```python
from build123d import *

# Parameters (mm, degrees)
F0_R     = 70
F1_DEPTH = 16
F2_R     = 31.12
F3_DEPTH = 16.001
F4_R     = 3.15
F4_R_2   = 8
F4_R_3   = 4
F5_DEPTH = 16.001
F6_R     = 45
F7_DEPTH = 2
F8_R     = 60
F8_R_2   = 58
F9_DEPTH = 2


with BuildPart() as f1:
    # F0 (on Top) → F1 (new body)
    with BuildSketch(Plane.XY):
        Circle(F0_R)
    extrude(amount=F1_DEPTH)

    # F2 (on face) → F3 (cut, through all)
    with BuildSketch(Plane.XY.offset(16)):
        Circle(F2_R)
    extrude(amount=-F3_DEPTH, mode=Mode.SUBTRACT)

    # F4 (on face) → F5 (cut, through all)
    with BuildSketch(Plane(origin=(0, 0, 0), x_dir=(1, 0, 0), z_dir=(0, 0, -1))):
        with BuildLine():
            Line((-19, -24.64659), (-19, -46.64659))
            ThreePointArc((-19, -46.64659), (0, -50.367692), (19, -46.64659))
            Line((19, -46.64659), (19, -24.64659))
            ThreePointArc((19, -24.64659), (0, -31.12), (-19, -24.64659))
        make_face()
        with Locations((-37.476659, -37.476659)):
            Circle(F4_R)
        with Locations((-45, 0)):
            Circle(F4_R_2)
        with Locations((-65, 0)):
            Circle(F4_R_3)
        with Locations((-37.476659, 37.476659)):
            Circle(F4_R)
        with Locations((37.476659, 37.476659)):
            Circle(F4_R)
        with Locations((37.476659, -37.476659)):
            Circle(F4_R)
        with Locations((65, 0)):
            Circle(F4_R_3)
        with Locations((0, 65)):
            Circle(F4_R_3)
        with Locations((0, -65)):
            Circle(F4_R_3)
    extrude(amount=-F5_DEPTH, mode=Mode.SUBTRACT)

    # F6 (on face) → F7 (cut)
    with BuildSketch(Plane(origin=(0, 0, 0), x_dir=(1, 0, 0), z_dir=(0, 0, -1))):
        Circle(F6_R)
    extrude(amount=-F7_DEPTH, mode=Mode.SUBTRACT)

    # F8 (on face) → F9 (cut)
    with BuildSketch(Plane(origin=(0, 0, 0), x_dir=(1, 0, 0), z_dir=(0, 0, -1))):
        Circle(F8_R)
        Circle(F8_R_2, mode=Mode.SUBTRACT)
    extrude(amount=-F9_DEPTH, mode=Mode.SUBTRACT)


solid = f1.part
```
For this review, take the finished solid that the model builds, in its own axes (mm). A direction names the side the tool comes from. Round coordinates to 2 decimals unless told otherwise and drop trailing zeros. Write each loop counter-clockwise with the first axis right and the second up, starting at its lowest first coordinate (ties: lowest second). Pieces come first, ordered by that corner, then holes. Notation, with made-up numbers: (-10.5, 23) - (0.5, 23) arc R10 ccw to (0.5, 29) - close; hole circle Ø1 at (-35, -33.5). An arc over 180 degrees is marked (long way). Put each result on its own line as item: value.
Q1. We need section D-D (x = 65). Give the boundary of the cut face in (y, z).
Solved:
outline: (-25.98, 0) - (-4, 0) - (-4, 16) - (-25.98, 16) - close; (4, 0) - (25.98, 0) - (25.98, 16) - (4, 16) - close
Q2. Mouldability with a two-part tool opening along X and no side actions: class faces 4 (the face through (-55.55, -42.594, 7.888)), 5 (the face through (-0.867, 68.905, 7.888)), 6 (the face through (15, -30, 16)) as released by +X, released by -X, zero draft, split by the parting line, or undercut.
Solved:
face 4: split by the parting line
face 5: undercut
face 6: zero draft
Q3. Machinability: for faces 1 (the face through (34, -30, 0)), 2 (the face through (-36, 27, 1)), 3 (the face through (-19, 35, 8)), which of the approach directions +Z, -Z, +X, -X, +Y, -Y give a long, thin tool a straight path to every point of the face, cutting with its end or side? Answer none if there is none.
Solved:
face 1: -Z, +X, -X, +Y, -Y
face 2: -Z
face 3: +Z, -Z
Q4. Wall thickness on probe 1 along Y at (x, z) = (0.5, 8.75); probe 2 along Y at (x, z) = (0, 0.9); probe 3 along X at (y, z) = (24, 1.5): over which ranges is each line inside the solid? List them lowest first.
Solved:
probe 1: y = -70 to -68.97, -61.03 to -31.12, 50.37 to 61.03, 68.97 to 70
probe 2: y = -70 to -69, -61 to -60, -58 to -45, 50.37 to 58, 60 to 61, 69 to 70
probe 3: x = -65.76 to -54.99, -52.8 to -38.07, 38.07 to 52.8, 54.99 to 65.76
Q5. We need section A-A (y = 0). Count the separate pieces of the cut face and the enclosed holes in it, and give its area (3 significant figures).
Solved:
separate pieces: 5
enclosed holes: 0
area: 685 mm2
Q6. We need section B-B (x = 0). Give the boundary of the cut face in (y, z).
Solved:
outline: (-70, 0) - (-69, 0) - (-69, 16) - (-70, 16) - close; (-61, 0) - (-60, 0) - (-60, 2) - (-58, 2) - (-58, 0) - (-45, 0) - (-45, 2) - (-31.12, 2) - (-31.12, 16) - (-61, 16) - close; (50.37, 0) - (58, 0) - (58, 2) - (60, 2) - (60, 0) - (61, 0) - (61, 16) - (50.37, 16) - close; (69, 0) - (70, 0) - (70, 16) - (69, 16) - close
Q7. Insertion check: pin 1 Ø7 at (x, y) = (0, -65) entering from -Z; pin 2 Ø5 at (x, z) = (22.5, 4) entering from +Y; pin 3 Ø8 at (x, z) = (16, 7.5) entering from -Y; pin 4 Ø4 at (y, z) = (36, 6) entering from +X. Each pin has a flat end and moves straight along its axis. Give the tip position at first contact, or say it passes through.
Solved:
pin 1: passes through
pin 2: stops at y = 67.08
pin 3: stops at y = -68.96
pin 4: stops at x = 61.19
